Work out the finished part from the listing and answer in its coordinate system (mm). A direction names the side the tool comes from. Give positions to 0.01 mm unless a question says otherwise; leave off trailing zeros. Loops run counter-clockwise (first coordinate to the right, second up) from the corner with the lowest first, then second, coordinate; pieces in that order, holes last. Notation, with made-up numbers: (40, 37.5) - (64, 37.5) arc R26 cw to (64, 53.5) - close; hole circle Ø2 at (-14.75, -26.75). An arc over 180 degrees is marked (long way). One line per question, with ' | ' between items. Start each with the question number.
1. Section D-D (y = 5.5) is taken. Determine the outline of the cut face in (x, z), plus the area to 3 significant figures.
2. Find the intervals of material crossed by line 1 (Z direction, x = 0, y = -4.5); line 2 (Y direction, x = 22.25, z = 3.75); line 3 (Z direction, x = -26, y = -5.75), in increasing order.
3. Which of the six approach directions +Z, -Z, +X, -X, +Y, -Y give full straight-line access (tool end or side, diameter ignored) to faces 1 (the face through (-2.17, -0.14, 21.24)), 2 (the face through (26, 0, 10.3)), 3 (the face through (-26, 0, 10.3))?
4. Section B-B (z = 31) is taken. Determine the outline of the cut face in (x, y).
5. Section A-A (y = 0) is taken. Determine the outline of the cut face in (x, z).
6. Each of these flat-tipped pins is pushed along its axis until it touches: pin 1 (4 mm diameter, centred on x = -22.25, y = 0, fed in from +Z); pin 2 (10 mm diameter, centred on y = -4, z = 39, fed in from +X); pin 3 (4.5 mm diameter, centred on x = 21, y = 1.5, fed in from +Z). Where does it stop, or does it pass through?
7. Section C-C (x = -22.25) is taken. Determine the outline of the cut face in (y, z), plus the area to 3 significant figures.
8. For a pull along X with two mould halves and no side action, classify faces 4 (the face through (18.803, 0.152, 5.078)), 5 (the face through (30.5, 0, 5)), 6 (the face through (0, -10, 20)) as released by +X, released by -X, zero draft, split by the parting line, or undercut.
from build123d import *

# Parameters (mm, degrees)
F1_DEPTH = 10
F2_R     = 10
F3_DEPTH = 10
F4_R     = 3.45
F5_DEPTH = 10.3


with BuildPart() as f1:
    # F0 (on Front) → F1 (new body, symmetric)
    with BuildSketch(Plane.XZ):
        Polygon((15.5, 51.5), (-15.5, 51.5), (-15.5, 10.3), (-30.5, 10.3), (-30.5, 0), (30.5, 0), (30.5, 10.3), (15.5, 10.3), align=None)
    extrude(amount=F1_DEPTH, both=True)

    # F2 (on Front) → F3 (cut, symmetric)
    with BuildSketch(Plane.XZ):
        with Locations((0, 31)):
            Circle(F2_R)
    extrude(amount=F3_DEPTH, both=True, mode=Mode.SUBTRACT)

    # F4 (on Top) → F5 (cut, through all)
    with BuildSketch(Plane.XY):
        with Locations((-22.25, 0)):
            Circle(F4_R)
        with Locations((22.25, 0)):
            Circle(F4_R)
    extrude(amount=F5_DEPTH, mode=Mode.SUBTRACT)


solid = f1.part
Conclusion:
1) outline: (-30.5, 0) - (30.5, 0) - (30.5, 10.3) - (15.5, 10.3) - (15.5, 51.5) - (-15.5, 51.5) - (-15.5, 10.3) - (-30.5, 10.3) - close; hole circle Ø20 at (0, 31) | area: 1,590 mm²
2) line 1: 0 to 21, 41 to 51.5 | line 2: -10 to -3.45, 3.45 to 10 | line 3: 0 to 10.3
3) face 1: +Y, -Y | face 2: +Z, +X, +Y, -Y | face 3: +Z, -X, +Y, -Y
4) outline: (-15.5, -10) - (-10, -10) - (-10, 10) - (-15.5, 10) - close; (10, -10) - (15.5, -10) - (15.5, 10) - (10, 10) - close
5) outline: (-30.5, 0) - (-25.7, 0) - (-25.7, 10.3) - (-30.5, 10.3) - close; (-18.8, 0) - (18.8, 0) - (18.8, 10.3) - (15.5, 10.3) - (15.5, 51.5) - (-15.5, 51.5) - (-15.5, 10.3) - (-18.8, 10.3) - close; (25.7, 0) - (30.5, 0) - (30.5, 10.3) - (25.7, 10.3) - close; hole circle Ø20 at (0, 31)
6) pin 1: through | pin 2: x = 15.5 | pin 3: z = 10.3
7) outline: (-10, 0) - (-3.45, 0) - (-3.45, 10.3) - (-10, 10.3) - close; (3.45, 0) - (10, 0) - (10, 10.3) - (3.45, 10.3) - close | area: 135 mm²
8) face 4: undercut | face 5: released by +X | face 6: zero draft
